from build123d import *

# Parameters (mm, degrees)
F0_R     = 12.7
F1_DEPTH = 6.35


with BuildPart() as f1:
    # F0 (on Top) → F1 (new body)
    with BuildSketch(Plane.XY):
        with BuildLine():
            ThreePointArc((-73.303587, -31.567672), (-60.319875, -33.890968), (-48.906375, -40.502055))
            ThreePointArc((-48.906375, -40.502055), (-45.783372, -43.442534), (-43.010688, -46.715423))
            ThreePointArc((-43.010688, -46.715423), (0, -63.5), (43.010688, -46.715423))
            ThreePointArc((43.010688, -46.715423), (45.783372, -43.442534), (48.906375, -40.502055))
            ThreePointArc((48.906375, -40.502055), (62.107619, -33.286067), (77.072974, -31.742878))
            ThreePointArc((77.072974, -31.742878), (108.150526, 0), (77.072974, 31.742878))
            ThreePointArc((77.072974, 31.742878), (75.049156, 31.602276), (73.020724, 31.569597))
            ThreePointArc((73.020724, 31.569597), (60.187156, 33.93985), (48.906375, 40.502055))
            ThreePointArc((48.906375, 40.502055), (45.783372, 43.442534), (43.010688, 46.715423))
            ThreePointArc((43.010688, 46.715423), (0, 63.5), (-43.010688, 46.715423))
            ThreePointArc((-43.010688, 46.715423), (-45.783372, 43.442534), (-48.906375, 40.502055))
            ThreePointArc((-48.906375, 40.502055), (-60.319875, 33.890968), (-73.303587, 31.567672))
            ThreePointArc((-73.303587, 31.567672), (-75.213159, 31.609643), (-77.118228, 31.747263))
            ThreePointArc((-77.118228, 31.747263), (-108.451321, 0), (-77.118228, -31.747263))
            ThreePointArc((-77.118228, -31.747263), (-75.213159, -31.609643), (-73.303587, -31.567672))
        make_face()
        with Locations((-76.701321, 0)):
            Circle(F0_R, mode=Mode.SUBTRACT)
        with BuildLine():
            ThreePointArc((-44.45, 0), (0, 44.45), (44.45, 0))
            ThreePointArc((44.45, 0), (0, -44.45), (-44.45, 0))
        make_face(mode=Mode.SUBTRACT)
        with Locations((76.400526, 0)):
            Circle(F0_R, mode=Mode.SUBTRACT)
    extrude(amount=F1_DEPTH)


solid = f1.part
The listing builds one solid part. Answer for the finished solid, in the listing's coordinates (mm). A direction names the side the tool comes from. Give positions to 0.01 mm unless a question says otherwise; leave off trailing zeros. Write each loop counter-clockwise with the first axis right and the second up, starting at its lowest first coordinate (ties: lowest second). Pieces come first, ordered by that corner, then holes. Notation, with made-up numbers: (-32, 33) -> (-20, 33) arc R29 ccw to (-20, 62) -> close; hole circle Ø8 at (-32, 26). An arc over 180 degrees is marked (long way). One line per question, with ' | ' between items. Start each with the question number.
1. Section A-A (y = 0) is taken. Determine the outline of the cut face in (x, z), plus the area to 3 significant figures.
2. Section D-D (y = -35) is taken. Determine the outline of the cut face in (x, z).
3. For a pull along Y with two mould halves and no side action, classify faces 1 (the cylindrical face through (-108.444, 0.692, 3.131)), 2 (the cylindrical face through (42.397, -13.352, 3.131)), 3 (the cylindrical face through (-75.24, -31.61, 3.13)) as pulls with the +Y half, pulls with the -Y half, needs draft (parallel to the pull), parting line crosses it, or undercut.
4. Section B-B (x = 0) is taken. Determine the outline of the cut face in (y, z), plus the area to 3 significant figures.
5. For faces 4 (the cylindrical face through (-75.19, 31.61, 3.13)), 5 (the cylindrical face through (-64.588, 3.815, 3.131)), determine the directions among +Z, -Z, +X, -X, +Y, -Y from which every point of the face is accessible in a straight line to the end or side of a thin tool.
6. Given pin 1 Ø23 at (x, y) = (76.4, 0) entering from -Z, flat-ended and moving along its own axis, determine where the tip first touches the part or whether it passes through.
7. Section C-C (z = 4.75) is taken. Determine the outline of the cut face in (x, y).
8. Find the intervals of material crossed by probe 1 along X at (y, z) = (-5.5, 2.25); probe 2 along Y at (x, z) = (-69.5, 4.75); probe 3 along X at (y, z) = (-9.5, 1.75), in increasing order.
Response values:
1) outline: (-108.45, 0) -> (-89.4, 0) -> (-89.4, 6.35) -> (-108.45, 6.35) -> close; (-64, 0) -> (-44.45, 0) -> (-44.45, 6.35) -> (-64, 6.35) -> close; (44.45, 0) -> (63.7, 0) -> (63.7, 6.35) -> (44.45, 6.35) -> close; (89.1, 0) -> (108.15, 0) -> (108.15, 6.35) -> (89.1, 6.35) -> close | area: 488 mm2
2) outline: (-57.62, 0) -> (-27.4, 0) -> (-27.4, 6.35) -> (-57.62, 6.35) -> close; (27.4, 0) -> (57.62, 0) -> (57.62, 6.35) -> (27.4, 6.35) -> close
3) face 1: parting line crosses it | face 2: undercut | face 3: pulls with the -Y half
4) outline: (-63.5, 0) -> (-44.45, 0) -> (-44.45, 6.35) -> (-63.5, 6.35) -> close; (44.45, 0) -> (63.5, 0) -> (63.5, 6.35) -> (44.45, 6.35) -> close | area: 242 mm2
5) face 4: +Z, -Z, +Y | face 5: +Z, -Z
6) pin 1: through
7) outline: (-77.12, -31.75) arc R38.1 cw to (-73.3, -31.57) arc R38.1 cw to (-48.91, -40.5) arc R38.1 cw to (-43.01, -46.72) arc R63.5 ccw to (43.01, -46.72) arc R38.1 cw to (48.91, -40.5) arc R38.1 cw to (77.07, -31.74) arc R31.75 ccw to (77.07, 31.74) arc R38.1 cw to (73.02, 31.57) arc R38.1 cw to (48.91, 40.5) arc R38.1 cw to (43.01, 46.72) arc R63.5 ccw to (-43.01, 46.72) arc R38.1 cw to (-48.91, 40.5) arc R38.1 cw to (-73.3, 31.57) arc R38.1 cw to (-77.12, 31.75) arc R31.75 ccw to start; hole circle Ø25.4 at (-76.7, 0); hole circle Ø88.9 at (0, 0); hole circle Ø25.4 at (76.4, 0)
8) probe 1: -107.97 to -88.15, -65.25 to -44.11, 44.11 to 64.95, 87.85 to 107.67 | probe 2: -31.77 to -10.46, 10.46 to 31.77 | probe 3: -107 to -85.13, -68.27 to -43.42, 43.42 to 67.97, 84.83 to 106.7
